Input: dimensioned drawing with shaded views. Units: mm. Origin: part minimum x, y, z. Give positions to 0.01 mm unless a question says otherwise; leave off trailing zeros. Order: outer loops, then holes, each group sorted by start corner. A loop starts at its lowest first (then second) coordinate and runs counter-clockwise, first axis right, second up.
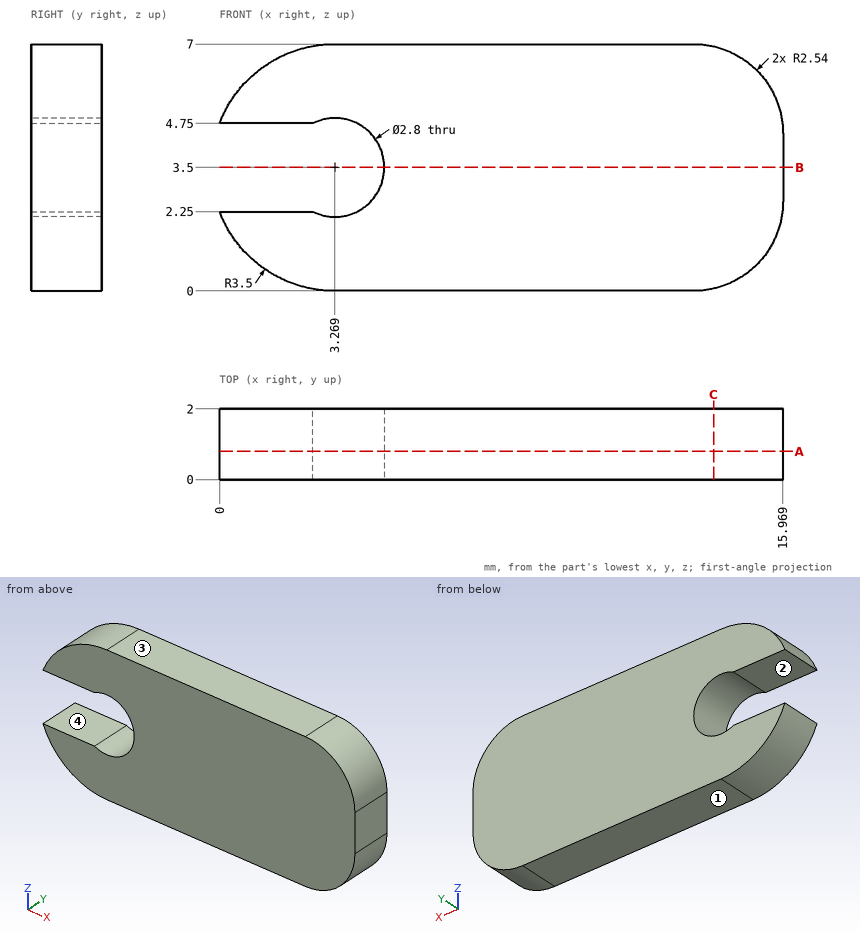
1) Draft query along Z for the marked faces 1, 2, 3 and 4. Return one class per face: +Z half, -Z half, draft (parallel to the pull), parting line (faces both ways), or undercut.
Report:
face 1: -Z half
face 2: undercut
face 3: +Z half
face 4: undercut
2) Material intervals for L1, parallel to X at y = 1, z = 3.5; L2, parallel to Z at x = 3, y = 1.5; L3, parallel to X at y = 0.75, z = 2.75, sorted ascending.
Report:
L1: x = 4.67 to 15.97
L2: z = 0.01 to 2.13, 4.87 to 6.99
L3: x = 4.45 to 15.97
3) Section query B-B, the plane z = 3.5. Return the cut outline in (x, y), and give its area (3 significant figures).
Report:
outline: (4.67, 0) - (15.97, 0) - (15.97, 2) - (4.67, 2) - close
area: 22.6 mm2
4) Section query A-A, the plane y = 0.8. Return the cut outline in (x, z), and give its area (3 significant figures).
Report:
outline: (0, 2.25) arc R3.5 ccw to (3.27, 0) - (13.43, 0) arc R2.54 ccw to (15.97, 2.54) - (15.97, 4.46) arc R2.54 ccw to (13.43, 7) - (3.27, 7) arc R3.5 ccw to (0, 4.75) - (2.64, 4.75) arc R1.4 cw (long way) to (2.64, 2.25) - close
area: 93.6 mm2
5) Section query C-C, the plane x = 14. Return the cut outline in (y, z) (3 decimals).
Report:
outline: (0, 0.065) - (2, 0.065) - (2, 6.935) - (0, 6.935) - close
6) Pin query (flat end, axial travel): pin 1 (3 mm diameter, centred on x = 9, z = 5, fed in from -Y). Return the tip coordinate at first contact, or that it passes through.
Report:
pin 1: stops at y = 0
